Could you check a few things on this model? Use its own coordinates, in mm. A direction names the side the tool comes from. Round coordinates to 2 decimals unless told otherwise and drop trailing zeros. Write each loop counter-clockwise with the first axis right and the second up, starting at its lowest first coordinate (ties: lowest second). Pieces come first, ordered by that corner, then holes. Notation, with made-up numbers: (3.5, 62) -> (15.5, 62) arc R27 ccw to (15.5, 90) -> close; hole circle Ø5 at (9.5, 60). An arc over 180 degrees is marked (long way). Return JSON: item names as keys, results as strings.
Autodesk Inventor part; units mm, degrees
ref_plane "YZ Plane" through (0, 0, 0) normal (1, 0, 0) x (0, 1, 0)
ref_plane "XZ Plane" through (0, 0, 0) normal (0, 1, 0) x (-1, 0, 0)
ref_plane "XY Plane" through (0, 0, 0) normal (0, 0, 1) x (1, 0, 0)
sketch "Sketch2" plane through (0, 0, 0) normal (0, 0, 1) x (1, 0, 0)
  line L0 (0, 0) -> (0, 6.5)
  line L1 (0, 6.5) -> (-2.5, 6.5) construction
  line L2 (-2.5, 6.5) -> (-2.5, 1)
  line L3 (-2.5, 1) -> (-2.75, 1)
  line L4 (-2.75, 1) -> (-2.75, 0)
  line L5 (-2.75, 0) -> (0, 0)
  arc A0 (0, 9) -> (-2.5, 6.5) centre (0, 6.5) ccw
  line L6 (0, 9) -> (0, 6.5)
  dimension "d11" = 5
  dimension "d12" = 5.5
  dimension "d13" = 5.5
  dimension "d14" = 1
revolve "Revolution1" add sketch "Sketch2" angle 360 about axis through (0, 0, 0) along (0, 1, 0)
sketch "Sketch3" plane through (0, 0, 0) normal (0, -1, 0) x (1, 0, 0)
  line L0 (-2.05, -0.35) -> (-1.35, -0.35)
  line L1 (-1.35, -0.35) -> (-1.35, 0.35)
  line L2 (-1.35, 0.35) -> (-2.05, 0.35)
  line L3 (-2.05, 0.35) -> (-2.05, -0.35)
  line L4 (-2.05, -0.35) -> (-1.35, 0.35) construction
  line L5 (-1.35, -0.35) -> (-2.05, 0.35) construction
  line L6 (1.35, -0.35) -> (2.05, -0.35)
  line L7 (2.05, -0.35) -> (2.05, 0.35)
  line L8 (2.05, 0.35) -> (1.35, 0.35)
  line L9 (1.35, 0.35) -> (1.35, -0.35)
  line L10 (1.35, -0.35) -> (2.05, 0.35) construction
  line L11 (2.05, -0.35) -> (1.35, 0.35) construction
  point P0 (0, 0)
  point P1 (-1.7, 0)
  point P2 (1.7, 0)
  point P3 (1.7, 0)
  dimension "d16" = 0.7
  dimension "d17" = 1.7
  dimension "d18" = 1.7
extrude "Extrusion2" add sketch "Sketch3" along normal blind 15
properties part number "P02 - LED 5mm" material "ABS Plastic"
1) I want a section at C-C, the plane z = 0. Please give me the cut outline in (x, y).
Return value:
{"outline": "(-2.75, 0) -> (-2.05, 0) -> (-2.05, -15) -> (-1.35, -15) -> (-1.35, 0) -> (1.35, 0) -> (1.35, -15) -> (2.05, -15) -> (2.05, 0) -> (2.75, 0) -> (2.75, 1) -> (2.5, 1) -> (2.5, 6.5) arc R2.5 ccw to (-2.5, 6.5) -> (-2.5, 1) -> (-2.75, 1) -> close"}
2) If I drill on probe 1 along X at (y, z) = (-0.5, -0.2); probe 2 along Z at (x, y) = (-1.7, -12); probe 3 along Y at (x, z) = (1.9, 1.9), over which ranges is the centre line in solid material (lowest first)? Write a range as [from, to].
Return value:
{"probe 1": "[-2.05, -1.35], [1.35, 2.05]", "probe 2": "[-0.35, 0.35]", "probe 3": "[0, 1]"}
3) For faces 1 (the face through (0.596, 0.493, 2.685)), 2 (the face through (0.54, 3.71, 2.44)), which set-ups out of +Z, -Z, +X, -X, +Y, -Y let a thin tool reach every point of the face, with its end or its side?
Return value:
{"face 1": "+Y, -Y", "face 2": "+Y"}
4) I want a section at A-A, the plane y = -3.5. Please give me the cut outline in (x, z), and give its area (3 significant figures).
Return value:
{"outline": "(-2.05, -0.35) -> (-1.35, -0.35) -> (-1.35, 0.35) -> (-2.05, 0.35) -> close; (1.35, -0.35) -> (2.05, -0.35) -> (2.05, 0.35) -> (1.35, 0.35) -> close", "area": "0.980 mm²"}
5) I want a section at B-B, the plane x = 0. Please give me the cut outline in (y, z), and give its area (3 significant figures).
Return value:
{"outline": "(0, -2.75) -> (1, -2.75) -> (1, -2.5) -> (6.5, -2.5) arc R2.5 ccw to (6.5, 2.5) -> (1, 2.5) -> (1, 2.75) -> (0, 2.75) -> close", "area": "42.8 mm²"}
6) I want a section at D-D, the plane y = 3.5. Please give me the cut outline in (x, z).
Return value:
{"outline": "circle Ø5 at (0, 0)"}
7) Will these pins go through, and if not, where does the flat tip stop? pin 1 Ø1 at (x, y) = (-2, 4) entering from +Z; pin 2 Ø1.5 at (y, z) = (4, -1.5) entering from +X; pin 3 Ø2 at (x, y) = (1.5, -12.5) entering from +Z.
Return value:
{"pin 1": "z = 2", "pin 2": "x = 2.38", "pin 3": "z = 0.35"}
